Can you work these out from the drawing? Everything is in mm from the part's minimum corner. Coordinates: 2 decimals unless noted, no trailing zeros. Order: outer loops, then holes, each group sorted by start corner. A loop starts at its lowest first (then second) coordinate and runs counter-clockwise, first axis right, second up. Notation, with made-up numbers: (-30.75, 57.5) - (18.25, 57.5) arc R14 ccw to (18.25, 75.5) - close; hole circle Ø8 at (51, 39). An arc over 180 degrees is marked (long way). Use a Markdown table: item, result. Add a question column.
(1) I want a section at C-C (x = 190.5). List the corners of the cut face in (y, z) for me (3 decimals), and give its area (3 significant figures).
(2) I want a section at D-D (z = 7). List the corners of the cut face in (x, y) for me, and give its area (3 significant figures).
(3) For pin 1 Ø1.5 at (y, z) = (3, 38.5) entering from +X; pin 2 Ø5.5 at (x, z) = (361.95, 25.4) entering from +Y; pin 3 Ø3 at (y, z) = (18.5, 44) entering from -X, each with a flat end and sliding along its axis, tell me the tip position at first contact or that it passes through.
(4) I want a section at A-A (z = 25.4). List the corners of the cut face in (x, y) for me (3 decimals), and give its area (3 significant figures).
(5) I want a section at B-B (y = 21). List the corners of the cut face in (x, z) for me (3 decimals).
(6) If I drill on L1, parallel to Z at x = 361.95, y = 8.75 (3 decimals); L2, parallel to X at y = 23.75, z = 25; L3, parallel to X at y = 21, z = 24, over which ranges is the centre line in solid material (lowest first)? Write a range as [from, to].
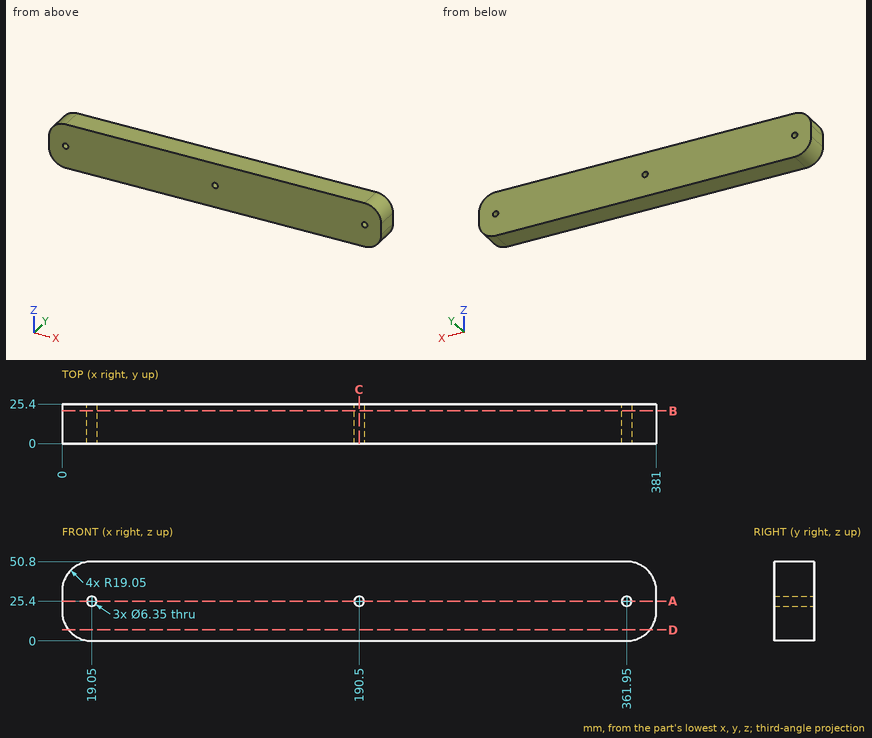
Answers follow:
| question | item | result |
|---|---|---|
| 1 | outline | (0, 0) - (25.4, 0) - (25.4, 22.225) - (0, 22.225) - close; (0, 28.575) - (25.4, 28.575) - (25.4, 50.8) - (0, 50.8) - close |
| 1 | area | 1,130 mm² |
| 2 | outline | (4.3, 0) - (376.7, 0) - (376.7, 25.4) - (4.3, 25.4) - close |
| 2 | area | 9,460 mm² |
| 3 | pin 1 | stops at x = 380.03 |
| 3 | pin 2 | passes through |
| 3 | pin 3 | stops at x = 3.32 |
| 4 | outline | (0, 0) - (15.875, 0) - (15.875, 25.4) - (0, 25.4) - close; (22.225, 0) - (187.325, 0) - (187.325, 25.4) - (22.225, 25.4) - close; (193.675, 0) - (358.775, 0) - (358.775, 25.4) - (193.675, 25.4) - close; (365.125, 0) - (381, 0) - (381, 25.4) - (365.125, 25.4) - close |
| 4 | area | 9,190 mm² |
| 5 | outline | (0, 19.05) arc R19.05 ccw to (19.05, 0) - (361.95, 0) arc R19.05 ccw to (381, 19.05) - (381, 31.75) arc R19.05 ccw to (361.95, 50.8) - (19.05, 50.8) arc R19.05 ccw to (0, 31.75) - close; hole circle Ø6.35 at (19.05, 25.4); hole circle Ø6.35 at (190.5, 25.4); hole circle Ø6.35 at (361.95, 25.4) |
| 6 | L1 | z = [0, 22.225], [28.575, 50.8] |
| 6 | L2 | x = [0, 15.9], [22.2, 187.35], [193.65, 358.8], [365.1, 381] |
| 6 | L3 | x = [0, 16.2], [21.9, 187.65], [193.35, 359.1], [364.8, 381] |
